Drawing for the job (mm, zero at the part's lowest x, y, z). A direction names the side the tool comes from. Coordinates: 2 decimals unless noted, no trailing zeros. Order: outer loops, then holes, each group sorted by start corner. A loop starts at its lowest first (then second) coordinate and runs counter-clockwise, first axis right, second up. Notation, with made-up numbers: (10.5, -22) - (18.5, -22) arc R20 cw to (18.5, 3) - close; hole circle Ø1 at (-15, 2). An arc over 180 degrees is marked (long way). Answer as CSV lines item,"result". Start each with the question number.
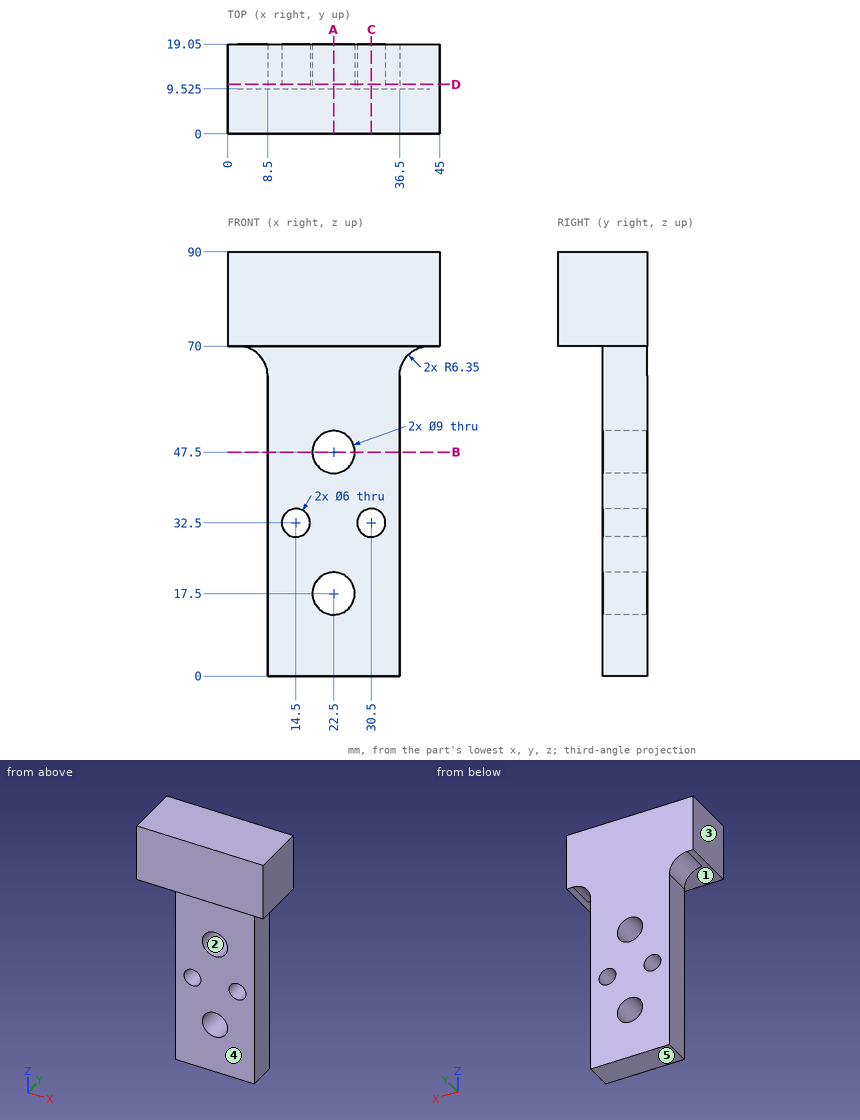
(1) Band-saw the part on B-B on z = 47.5. List the corners of the cut face in (x, y) (3 decimals), plus the area to 3 significant figures.
(2) Band-saw the part on C-C on x = 30.5. List the corners of the cut face in (y, z) (3 decimals).
(3) Band-saw the part on D-D on y = 10.5. List the corners of the cut face in (x, z), plus the area to 3 significant figures.
(4) Drop flat-ended pins along their axis: pin 1 Ø1 at (x, z) = (12, 68.5) entering from -Y (3 decimals); pin 2 Ø7.5 at (y, z) = (13.5, 33) entering from -X; pin 3 Ø3 at (y, z) = (14.5, 22.5) entering from +X. Give the stop position or say it passes through.
(5) Probe L1, parallel to Z at x = 22.5, y = 16.25; L2, parallel to X at y = 17, z = 30.5; L3, parallel to Z at x = 30.5, y = 14.25. List the from-to ranges inside material, lowest first. Write a range as [from, to].
(6) Band-saw the part on A-A on x = 22.5. List the corners of the cut face in (y, z) (3 decimals).
(7) Which spindle directions (+Z, -Z, +X, -X, +Y, -Y) get a long thin tool onto all of the face, cutting with end or side? Do the marked faces 4 and 5. Say none if no direction does.
(8) Pull direction X, two halves, no side cores. Call the marked faces 1, 2 and 3: +X half, -X half, draft (parallel to the pull), parting line (faces both ways), or undercut.
Filled in:
1,outline,"(8.5, 9.525) - (18, 9.525) - (18, 19.05) - (8.5, 19.05) - close; (27, 9.525) - (36.5, 9.525) - (36.5, 19.05) - (27, 19.05) - close"
1,area,"181 mm^2"
2,outline,"(0, 70) - (9.525, 70) - (9.525, 35.5) - (19.05, 35.5) - (19.05, 90) - (0, 90) - close; (9.525, 0) - (19.05, 0) - (19.05, 29.5) - (9.525, 29.5) - close"
3,outline,"(0, 70) - (2.15, 70) arc R6.35 cw to (8.5, 63.65) - (8.5, 0) - (36.5, 0) - (36.5, 63.65) arc R6.35 cw to (42.85, 70) - (45, 70) - (45, 90) - (0, 90) - close; hole circle Ø6 at (14.5, 32.5); hole circle Ø9 at (22.5, 17.5); hole circle Ø9 at (22.5, 47.5); hole circle Ø6 at (30.5, 32.5)"
3,area,"2,690 mm^2"
4,pin 1,"stops at y = 9.525"
4,pin 2,"stops at x = 8.5"
4,pin 3,"stops at x = 36.5"
5,L1,"z = [0, 13], [22, 43], [52, 90]"
5,L2,"x = [8.5, 12.26], [16.74, 28.26], [32.74, 36.5]"
5,L3,"z = [0, 29.5], [35.5, 90]"
6,outline,"(0, 70) - (9.525, 70) - (9.525, 52) - (19.05, 52) - (19.05, 90) - (0, 90) - close; (9.525, 0) - (19.05, 0) - (19.05, 13) - (9.525, 13) - close; (9.525, 22) - (19.05, 22) - (19.05, 43) - (9.525, 43) - close"
7,face 4,"-Z, +X, -X, -Y"
7,face 5,"-Z, +X, -X, +Y, -Y"
8,face 1,"draft"
8,face 2,"undercut"
8,face 3,"-X half"
